Read the model definition and answer for the solid it produces. Units are mm, in the model's axes. Face numbers are marked on the shaded views. A direction names the side the tool comes from. Give positions to 0.01 mm unless a question says otherwise; leave off trailing zeros. Write each loop counter-clockwise with the first axis right and the second up, starting at its lowest first coordinate (ties: lowest second). Pieces come first, ordered by that corner, then holes. Notation, with made-up numbers: (-13, 68.5) - (-2, 68.5) arc R27 cw to (-2, 107.5) - close; hole circle Ø7 at (22, 67.25). An arc over 180 degrees is marked (long way). Answer as CSV lines item,"result".
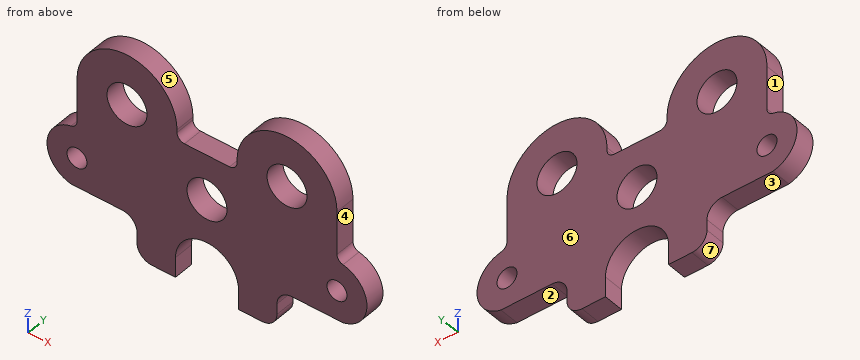
```python
from build123d import *

# Parameters (mm, degrees)
F0_R     = 6.35
F0_R_2   = 12.7
F1_DEPTH = 12.7


with BuildPart() as f1:
    # F0 (on Front) → F1 (new body)
    with BuildSketch(Plane.XZ):
        with BuildLine():
            Line((4.658427, 38.324708), (-23.916573, 38.324708))
            ThreePointArc((-23.916573, 38.324708), (-27.284169, 39.719612), (-28.679073, 43.087208))
            Line((-28.679073, 43.087208), (-28.679073, 44.898387))
            ThreePointArc((-28.679073, 44.898387), (-60.541307, 76.648584), (-92.179073, 44.674708))
            Line((-92.179073, 44.674708), (-92.179073, 17.206098))
            ThreePointArc((-92.179073, 17.206098), (-93.252557, 14.194029), (-95.989073, 12.53982))
            ThreePointArc((-95.989073, 12.53982), (-111.229073, -6.125292), (-95.989073, -24.790403))
            Line((-95.989073, -24.790403), (-92.179073, -24.790403))
            Line((-92.179073, -24.790403), (-63.604073, -24.790403))
            ThreePointArc((-63.604073, -24.790403), (-56.868881, -27.580211), (-54.079073, -34.315403))
            Line((-54.079073, -34.315403), (-54.079073, -41.050292))
            ThreePointArc((-54.079073, -41.050292), (-51.289266, -47.785484), (-44.554073, -50.575292))
            Line((-44.554073, -50.575292), (-29.646001, -50.575292))
            Line((-29.646001, -50.575292), (-29.646001, -37.875292))
            ThreePointArc((-29.646001, -37.875292), (-9.629073, -17.858364), (10.387854, -37.875292))
            Line((10.387854, -37.875292), (10.387854, -50.575292))
            Line((10.387854, -50.575292), (25.295927, -50.575292))
            ThreePointArc((25.295927, -50.575292), (32.031119, -47.785484), (34.820927, -41.050292))
            Line((34.820927, -41.050292), (34.820927, -34.315403))
            ThreePointArc((34.820927, -34.315403), (37.610734, -27.580211), (44.345927, -24.790403))
            Line((44.345927, -24.790403), (72.920927, -24.790403))
            Line((72.920927, -24.790403), (76.730927, -24.790403))
            ThreePointArc((76.730927, -24.790403), (91.970927, -6.125292), (76.730927, 12.53982))
            ThreePointArc((76.730927, 12.53982), (73.99441, 14.194029), (72.920927, 17.206098))
            Line((72.920927, 17.206098), (72.920927, 44.674708))
            ThreePointArc((72.920927, 44.674708), (41.28316, 76.648584), (9.420927, 44.898387))
            Line((9.420927, 44.898387), (9.420927, 43.087208))
            ThreePointArc((9.420927, 43.087208), (8.026023, 39.719612), (4.658427, 38.324708))
        make_face()
        with Locations((-92.179073, -6.125292)):
            Circle(F0_R, mode=Mode.SUBTRACT)
        with Locations((-9.629073, 9.749708)):
            Circle(F0_R_2, mode=Mode.SUBTRACT)
        with Locations((72.920927, -6.125292)):
            Circle(F0_R, mode=Mode.SUBTRACT)
        with Locations((-60.429073, 44.674708)):
            Circle(F0_R_2, mode=Mode.SUBTRACT)
        with Locations((41.170927, 44.674708)):
            Circle(F0_R_2, mode=Mode.SUBTRACT)
    extrude(amount=F1_DEPTH)


solid = f1.part
```
(1) A cutting plane is placed at B-B (z = 68.5). Write down the section's boundary in (x, y).
Worked out:
outline,"(-81.67, -12.7) - (-39.19, -12.7) - (-39.19, 0) - (-81.67, 0) - close; (19.93, -12.7) - (62.41, -12.7) - (62.41, 0) - (19.93, 0) - close"
(2) A cutting plane is placed at A-A (x = -18). Write down the section's boundary in (y, z).
Worked out:
outline,"(-12.7, -19.69) - (0, -19.69) - (0, 0.2) - (-12.7, 0.2) - close; (-12.7, 19.3) - (0, 19.3) - (0, 38.32) - (-12.7, 38.32) - close"
(3) A cutting plane is placed at C-C (y = -6.5). Count the separate pieces of the cut face and the enclosed holes in it, and give its area (3 significant figures).
Worked out:
separate pieces,"1"
enclosed holes,"5"
area,"15,000 mm^2"
(4) Each of these flat-tipped pins is pushed along its axis until it touches: P1, Ø4, axis at y = -4, z = -41, coming from the +X side; P2, Ø2, axis at y = -5.5, z = 43.5, coming from the -X side; P3, Ø1.5, axis at x = -26, y = -1.5, coming from the +Z side; P4, Ø7.5, axis at x = -92.18, z = -6.13, coming from the -Y side. Where does it stop, or does it pass through?
Worked out:
P1,"stops at x = 34.82"
P2,"stops at x = -92.18"
P3,"stops at z = 39.26"
P4,"passes through"
(5) For the marked faces 1, 2 and 3, determine the directions among +Z, -Z, +X, -X, +Y, -Y from which every point of the face is accessible in a straight line to the end or side of a thin tool.
Worked out:
face 1,"+Z, -X, +Y, -Y"
face 2,"-Z, +X, +Y, -Y"
face 3,"-Z, -X, +Y, -Y"
(6) The mould has two halves that part along X. Classify the marked faces 4, 5, 6 and 7: +X half, -X half, draft (parallel to the pull), parting line (faces both ways), or undercut.
Worked out:
face 4,"+X half"
face 5,"undercut"
face 6,"draft"
face 7,"-X half"
(7) Find the intervals of material crossed by L1, parallel to X at y = -12, z = 45; L2, parallel to X at y = -5.5, z = -40; L3, parallel to X at y = -1.25, z = 33.5, in increasing order.
Worked out:
L1,"x = -92.18 to -73.12, -47.73 to -28.68, 9.42 to 28.48, 53.87 to 72.92"
L2,"x = -54.08 to -29.65, 10.39 to 34.82"
L3,"x = -92.18 to -66.46, -54.39 to 35.14, 47.21 to 72.92"
(8) A cutting plane is placed at D-D (x = -79). Write down the section's boundary in (y, z), and give its area (3 significant figures).
Worked out:
outline,"(-12.7, -24.79) - (0, -24.79) - (0, 70.65) - (-12.7, 70.65) - close"
area,"1,210 mm^2"
